Design review of the part built by this model. Coordinates are the model's own, in mm. A direction names the side the tool comes from. Coordinates: 2 decimals unless noted, no trailing zeros. Write each loop counter-clockwise with the first axis right and the second up, starting at its lowest first coordinate (ties: lowest second). Pieces come first, ordered by that corner, then holes. Notation, with made-up numbers: M 31,-33.5 L 90,-33.5 A22 ccw 90,-27.5 Z; hole C 18.25,39.5 d2. An arc over 180 degrees is marked long. Write item = value, one per line.
```python
from build123d import *

# Parameters (mm, degrees)
SKETCH_1_W          = 120
SKETCH_1_H          = 34
EXTRUDE_1_DEPTH     = 3
SKETCH_2_R          = 1.25
CUT_EXTRUDE_1_DEPTH = 63.433965115
SKETCH_2_3_R        = 2
CUT_EXTRUDE_2_DEPTH = 1.5
SKETCH_3_R          = 0.35
CUT_EXTRUDE_3_DEPTH = 3
SKETCH_4_R          = 0.35
CUT_EXTRUDE_4_DEPTH = 3


with BuildPart() as part:
    # Sketch 1 → Extrude 1 (new body)
    with BuildSketch(Plane(origin=(0, 0, 0), x_dir=(1, 0, 0), z_dir=(0, 1, 0))):
        Rectangle(SKETCH_1_W, SKETCH_1_H)
    extrude(amount=EXTRUDE_1_DEPTH)

    # Sketch 2 → Cut-Extrude 1 (cut, through all)
    with BuildSketch(Plane(origin=(0, 3, 0), x_dir=(1, 0, 0), z_dir=(0, 1, 0))):
        with Locations(Location((-24.857141963, 14.500000041, 0), (0, 0, 270))):
            Circle(SKETCH_2_R)
        with Locations(Location((27.857143751, 14.500000041, 0), (0, 0, 270))):
            Circle(SKETCH_2_R)
    extrude(amount=-CUT_EXTRUDE_1_DEPTH, mode=Mode.SUBTRACT)

    # Sketch 2_3 → Cut-Extrude 2 (cut)
    with BuildSketch(Plane(origin=(0, 3, 0), x_dir=(1, 0, 0), z_dir=(0, 1, 0))):
        with Locations(Location((-24.857141963, 14.500000041, 0), (0, 0, 270))):
            Circle(SKETCH_2_3_R)
        with Locations(Location((27.857143751, 14.500000041, 0), (0, 0, 270))):
            Circle(SKETCH_2_3_R)
    extrude(amount=-CUT_EXTRUDE_2_DEPTH, mode=Mode.SUBTRACT)

    # Sketch 3 → Cut-Extrude 3 (cut)
    with BuildSketch(Plane(origin=(60, 0, 0), x_dir=(0, 0, -1), z_dir=(1, 0, 0))):
        with Locations((-8.5, 1.5)):
            Circle(SKETCH_3_R)
        with Locations((8.5, 1.5)):
            Circle(SKETCH_3_R)
    extrude(amount=-CUT_EXTRUDE_3_DEPTH, mode=Mode.SUBTRACT)

    # Sketch 4 → Cut-Extrude 4 (cut)
    with BuildSketch(Plane.XY.offset(17)):
        with Locations((-29.25, 1.5)):
            Circle(SKETCH_4_R)
        with Locations((1.5, 1.5)):
            Circle(SKETCH_4_R)
        with Locations((32.25, 1.5)):
            Circle(SKETCH_4_R)
    extrude(amount=-CUT_EXTRUDE_4_DEPTH, mode=Mode.SUBTRACT)


solid = part.part
```
Q1. Wall thickness on line 1 (X direction, y = 1.45, z = 14.5); line 2 (X direction, y = 1.2, z = -14.5); line 3 (Y direction, x = 32.25, z = 16.3): over which ranges is each line inside the solid? List them lowest first.
Check result:
line_1 = -60 to -29.6, -28.9 to 1.15, 1.85 to 31.9, 32.6 to 60
line_2 = -60 to -26.11, -23.61 to 26.61, 29.11 to 60
line_3 = 0 to 1.15, 1.85 to 3
Q2. For P1, Ø3.5, axis at x = 27.86, z = -14.5, coming from the +Y side; P2, Ø0.8, axis at x = -29.5, y = 1.5, coming from the +Z side; P3, Ø2, axis at x = -24.86, z = -14.5, coming from the +Y side; P4, Ø0.6, axis at x = 1.5, y = 1.5, coming from the +Z side, all flat-tipped, find the tip position at first contact; note any pin that passes through.
Check result:
P1 = 1.5
P2 = 17
P3 = through
P4 = 14
Q3. Consider section A-A, the plane z = -14.5. State the section outline as (x, y) points, and give its area (4 significant figures).
Check result:
outline = M -60,0 L -26.11,0 L -26.11,1.5 L -26.86,1.5 L -26.86,3 L -60,3 Z; M -23.61,0 L 26.61,0 L 26.61,1.5 L 25.86,1.5 L 25.86,3 L -22.86,3 L -22.86,1.5 L -23.61,1.5 Z; M 29.11,0 L 60,0 L 60,3 L 29.86,3 L 29.86,1.5 L 29.11,1.5 Z
area = 340.5 mm²
Q4. Machinability: for faces 1 (the cylindrical face through (26.637, 0.76, -14.771)), 2 (the flat face through (-25, 1.5, -13)), which of the approach directions +Z, -Z, +X, -X, +Y, -Y give a long, thin tool a straight path to every point of the face, cutting with its end or side? Answer none if there is none.
Check result:
face_1 = +Y, -Y
face_2 = +Y
Q5. The part is to be moulded in two halves that separate along X. For faces 3 (the cylindrical face through (29.84, 2.26, -14.76)), 4 (the flat face through (-1, 1, -17)), 5 (the flat face through (-60, 1, 0)), say which applies: +X half, -X half, draft (parallel to the pull), parting line (faces both ways), or undercut.
Check result:
face_3 = undercut
face_4 = draft
face_5 = -X half
